Source: CAD feature listing. Evaluate the final solid. Frame: model axes, mm. Face numbers are marked on the shaded views. A direction names the side the tool comes from. Round coordinates to 2 decimals unless told otherwise and drop trailing zeros. Order: outer loops, then holes, each group sorted by start corner. A loop starts at its lowest first (then second) coordinate and runs counter-clockwise, first axis right, second up. Notation, with made-up numbers: M -39,70 L 17,70 A16 cw 17,79 Z; hole C 14,51 d6. An arc over 180 degrees is marked long. Use CSV: the item, a comma, the result in double quotes. Start each with the question number.
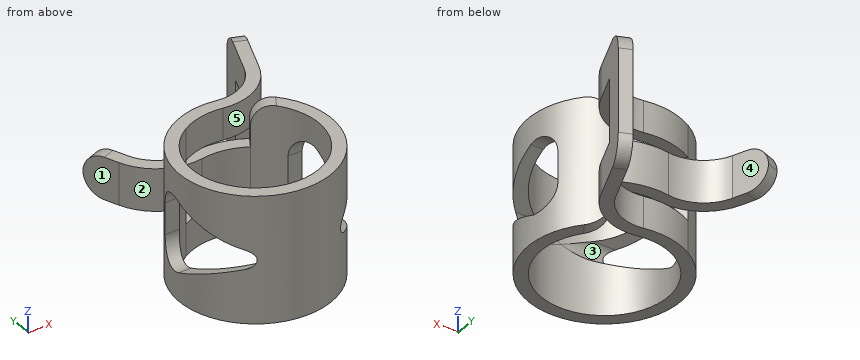
```python
from build123d import *

# Parameters (mm, degrees)
CYLINDER_SKETCH_R               = 3.6
CYLINDER_SKETCH_R_2             = 3
CYLINDER_EXTRUDE_DEPTH          = 3
CUT_SIDE_SLOTS_DEPTH            = 12.7
CUT_SLOT_IN_TOP_DEPTH           = 8.868926397
FEMALE_BASE_SKETCH_W            = 1.5
FEMALE_BASE_SKETCH_H            = 0.6
FEMALE_BASE_ANGLE               = 40.5
FEMALE_TRANSITION_SKETCH_W      = 1.5
FEMALE_TRANSITION_SKETCH_H      = 0.6
FEMALE_TRANSITION_REVOLVE_ANGLE = 78
FEMALE_LEVER_SKETCH_W           = 0.6
FEMALE_LEVER_SKETCH_H           = 1.5
FEMALE_LEVER_EXTRUDE_DEPTH      = 1.5
FEMALE_TOP_SKETCH_W             = 0.6
FEMALE_TOP_SKETCH_H             = 6
FEMALE_TOP_EXTRUDE_DEPTH        = 1.5
MALE_BASE_SKETCH_W              = 2
MALE_BASE_SKETCH_H              = 0.6
MALE_BASE_ANGLE                 = 40.5
MALE_TRANSITION_SKETCH_W        = 2
MALE_TRANSITION_SKETCH_H        = 0.6
MALE_TRANSITION_REVOLVE_ANGLE   = 78
MALE_LEVER_SKETCH_W             = 0.6
MALE_LEVER_SKETCH_H             = 2
MALE_LEVER_EXTRUDE_DEPTH        = 1.714285714
FILLETS_R                       = 1.016


with BuildPart() as part:
    # Cylinder Sketch → Cylinder Extrude (new, symmetric)
    with BuildSketch(Plane.XY):
        Circle(CYLINDER_SKETCH_R)
        Circle(CYLINDER_SKETCH_R_2, mode=Mode.SUBTRACT)
    extrude(amount=CYLINDER_EXTRUDE_DEPTH, both=True)

    # Side Slot Sketch → Cut Side Slots (cut, symmetric)
    with BuildSketch(Plane(origin=(0, 0, 0), x_dir=(0, 0, -1), z_dir=(1, 0, 0))):
        with BuildLine():
            Line((-0.75, 1.5), (0.75, 1.5))
            ThreePointArc((0.75, 1.5), (1.585525874, 1.049451102), (1.668161225, 0.103793027))
            Line((1.668161225, 0.103793027), (0.459080612, -2.698103486))
            ThreePointArc((0.459080612, -2.698103486), (0, -3), (-0.459080612, -2.698103486))
            Line((-0.459080612, -2.698103486), (-1.668161225, 0.103793027))
            ThreePointArc((-1.668161225, 0.103793027), (-1.585525874, 1.049451102), (-0.75, 1.5))
        make_face()
    extrude(amount=CUT_SIDE_SLOTS_DEPTH, both=True, mode=Mode.SUBTRACT)

    # Top Slot Sketch → Cut Slot in Top (cut, through all)
    with BuildSketch(Plane.XY.offset(3)):
        Polygon((-2.163098228, 3.6), (0, 0), (2.163098228, 3.6), align=None)
    extrude(amount=-CUT_SLOT_IN_TOP_DEPTH, mode=Mode.SUBTRACT)

    # Female Base Sketch → Female Base (revolve)
    with BuildSketch(Plane(origin=(0, 0, 0), x_dir=(0, 0, -1), z_dir=(0.8571673007021136, 0.515038074910052, 0))):
        with Locations((-2.25, 3.3)):
            Rectangle(FEMALE_BASE_SKETCH_W, FEMALE_BASE_SKETCH_H)
        with Locations((2.25, 3.3)):
            Rectangle(FEMALE_BASE_SKETCH_W, FEMALE_BASE_SKETCH_H)
    revolve(axis=Axis((0, 0, 0), (0, 0, -1)), revolution_arc=FEMALE_BASE_ANGLE)

    # Female Transition Sketch → Female Transition Revolve (revolve)
    with BuildSketch(Plane(origin=(0, 0, 0), x_dir=(0, 0, -1), z_dir=(0.9862856015372308, -0.16504760586068196, 0))):
        with Locations((2.25, 3.3)):
            Rectangle(FEMALE_TRANSITION_SKETCH_W, FEMALE_TRANSITION_SKETCH_H)
        with Locations((-2.25, 3.3)):
            Rectangle(FEMALE_TRANSITION_SKETCH_W, FEMALE_TRANSITION_SKETCH_H)
    revolve(axis=Axis((0.924266593, 5.523199369, 1.5), (0, 0, 1)), revolution_arc=FEMALE_TRANSITION_REVOLVE_ANGLE)

    # Female Lever Sketch → Female Lever Extrude (add)
    with BuildSketch(Plane(origin=(2.007556855, 5.096479986, 0), x_dir=(0.9304175679820241, -0.3665012267242986, 0), z_dir=(0.3665012267242986, 0.9304175679820241, 0))):
        with Locations((1.135694531, 2.25)):
            Rectangle(FEMALE_LEVER_SKETCH_W, FEMALE_LEVER_SKETCH_H)
        with Locations((1.135694531, -2.25)):
            Rectangle(FEMALE_LEVER_SKETCH_W, FEMALE_LEVER_SKETCH_H)
    extrude(amount=FEMALE_LEVER_EXTRUDE_DEPTH)

    # Female Top Sketch → Female Top Extrude (add)
    with BuildSketch(Plane(origin=(2.557308695, 6.492106338, 0), x_dir=(0.930417567982024, -0.3665012267242986, 0), z_dir=(0.3665012267242986, 0.9304175679820241, 0))):
        with Locations((1.135694531, 0)):
            Rectangle(FEMALE_TOP_SKETCH_W, FEMALE_TOP_SKETCH_H)
    extrude(amount=FEMALE_TOP_EXTRUDE_DEPTH)

    # Male Base Sketch → Male Base (revolve)
    with BuildSketch(Plane(origin=(0, 0, 0), x_dir=(0, 0, 1), z_dir=(-0.8571673007021136, 0.515038074910052, 0))):
        with Locations((0, 3.3)):
            Rectangle(MALE_BASE_SKETCH_W, MALE_BASE_SKETCH_H)
    revolve(axis=Axis((0, 0, 0), (0, 0, 1)), revolution_arc=MALE_BASE_ANGLE)

    # Male Transition Sketch → Male Transition Revolve (revolve)
    with BuildSketch(Plane(origin=(0, 0, 0), x_dir=(0, 0, 1), z_dir=(-0.9862856015372308, -0.16504760586068182, 0))):
        with Locations((0, 3.3)):
            Rectangle(MALE_TRANSITION_SKETCH_W, MALE_TRANSITION_SKETCH_H)
    revolve(axis=Axis((-0.924266593, 5.523199369, -1), (0, 0, -1)), revolution_arc=MALE_TRANSITION_REVOLVE_ANGLE)

    # Male Lever Sketch → Male Lever Extrude (add)
    with BuildSketch(Plane(origin=(-2.007556855, 5.096479986, 0), x_dir=(0.9304175679820241, 0.3665012267242986, 0), z_dir=(-0.3665012267242986, 0.9304175679820241, 0))):
        with Locations((-1.135694531, 0)):
            Rectangle(MALE_LEVER_SKETCH_W, MALE_LEVER_SKETCH_H)
    extrude(amount=MALE_LEVER_EXTRUDE_DEPTH)

    # Fillets
    # the kernel refuses this fillet: 1.016 mm, written as the material it takes off along each edge
    with BuildSketch(Plane(origin=(0.236917514, 0.394296958, -3), x_dir=(0.8571673007021136, -0.5150380749100519, 0), z_dir=(0.515038074910052, 0.8571673007021137, 0))) as fillets_piece_1_section:
        with BuildLine():
            CenterArc((FILLETS_R, -FILLETS_R), FILLETS_R, 90, 90)
            Line((0, -FILLETS_R), (0, 0))
            Line((0, 0), (FILLETS_R, 0))
        make_face()
    fillets_piece_1 = extrude(amount=5.68, mode=Mode.PRIVATE)
    fillets_piece_1 = fillets_piece_1 & Plane(origin=(0, 0, -2.773460416), x_dir=(1, 0, 0), z_dir=(0, 0, 1)) * Cylinder(3.6, 16, mode=Mode.PRIVATE)
    add(fillets_piece_1, mode=Mode.SUBTRACT)
    with BuildSketch(Plane(origin=(0.236917514, 0.394296958, 3), x_dir=(0, 0, -1), z_dir=(0.515038074910052, 0.8571673007021137, 0))) as fillets_piece_2_section:
        with BuildLine():
            CenterArc((FILLETS_R, -FILLETS_R), FILLETS_R, 90, 90)
            Line((0, -FILLETS_R), (0, 0))
            Line((0, 0), (FILLETS_R, 0))
        make_face()
    fillets_piece_2 = extrude(amount=5.68, mode=Mode.PRIVATE)
    fillets_piece_2 = fillets_piece_2 & Plane(origin=(0, 0, 2.773461153), x_dir=(1, 0, 0), z_dir=(0, 0, 1)) * Cylinder(3.6, 16, mode=Mode.PRIVATE)
    add(fillets_piece_2, mode=Mode.SUBTRACT)
    with BuildSketch(Plane(origin=(-6.334900709, 5.234384608, 1), x_dir=(0.3665012267242986, -0.930417567982024, 0), z_dir=(0.9304175679820241, 0.3665012267242986, 0)), Plane(origin=(-1.050128923, 7.316111576, -1), x_dir=(0.3665012267242985, -0.930417567982024, 0), z_dir=(-0.9304175679820241, -0.3665012267242986, 0))) as fillets_piece_3:
        with BuildLine():
            CenterArc((FILLETS_R, FILLETS_R), FILLETS_R, 180, 90)
            Line((0, FILLETS_R), (0, 0))
            Line((0, 0), (FILLETS_R, 0))
        make_face()
    extrude(amount=5.68, mode=Mode.SUBTRACT)
    with BuildSketch(Plane(origin=(1.521344786, 8.512362735, -3), x_dir=(-0.3665012267242986, -0.930417567982024, 0), z_dir=(0.9304175679820241, -0.3665012267242986, 0)), Plane(origin=(6.806116572, 6.430635767, 3), x_dir=(-0.3665012267242985, -0.930417567982024, 0), z_dir=(-0.9304175679820241, 0.3665012267242986, 0))) as fillets_piece_4:
        with BuildLine():
            CenterArc((FILLETS_R, -FILLETS_R), FILLETS_R, 90, 90)
            Line((0, -FILLETS_R), (0, 0))
            Line((0, 0), (FILLETS_R, 0))
        make_face()
    extrude(amount=5.68, mode=Mode.SUBTRACT)


solid = part.part
```
(1) Reachability of the marked faces 3, 4 and 5 from +Z, -Z, +X, -X, +Y, -Y: full face, straight path, thin tool, end or side. Return the list, or none.
(2) Line query: line 1 along Y through (x, z) = (2, -2.25); line 2 along Y through (x, z) = (0, -0.25); line 3 along Y through (x, z) = (0, 1.25). Output: solid intervals per line, ascending.
(3) Section B-B on z = -1.25. Return loops of the section in (x, y).
(4) Section A-A on x = -0.25. Return loops of the section in (y, z).
(5) Section C-C on x = -2. Return loops of the section in (y, z).
(6) Draft query along Z for the marked faces 1 and 2. Return one class per face: pulls with the +Z half, pulls with the -Z half, needs draft (parallel to the pull), parting line crosses it, or undercut.
(7) Contact query for flat-ended pins moving along their axis: P1, Ø3.5, axis at x = 0, y = 0, coming from the +Z side; P2, Ø2, axis at y = -1, z = -2, coming from the -X side; P3, Ø2, axis at x = 3, z = 0.5, coming from the -Y side. Output: stop coordinate, or through.
Results below:
1,face 3,"+X, -X"
1,face 4,"+Z, -Z, +Y"
1,face 5,"+Z"
2,line 1,"y = -2.99 to -2.24, 2.24 to 2.99, 3.16 to 3.84"
2,line 2,"y = -3.6 to -3, 3 to 3.6"
2,line 3,"y = -3.6 to -3"
3,outline,"M -3.49,-0.87 A3.6 ccw 3.49,-0.87 L 2.87,-0.87 A3 cw -2.87,-0.87 Z; M -3.33,1.37 L -2.67,1.37 A3 cw -1.55,2.57 L -1.85,3.09 A3.6 ccw Z; M 1.55,2.57 A3 cw 2.67,1.37 L 3.33,1.37 A3.6 ccw 1.85,3.09 Z; M 3.33,6.19 L 3.89,5.97 L 4.44,7.36 L 3.88,7.58 Z"
4,outline,"M -3.59,-3 L -2.99,-3 L -2.99,-0.1 A0.5 cw -2.99,0.1 L -2.99,3 L -3.59,3 Z; M 2.99,-3 L 3.59,-3 L 3.59,-1.5 L 2.99,-1.5 Z; M 2.99,-1 L 3.59,-1 L 3.59,1 L 2.99,1 Z; M 2.99,1.5 L 3.59,1.5 L 3.59,3 L 2.99,3 Z"
5,outline,"M -2.99,-3 L -2.24,-3 L -2.24,-0.66 L -2.7,-0.46 A0.5 cw -2.99,-0.08 Z; M -2.99,0.08 A0.5 cw -2.7,0.46 L -2.24,0.66 L -2.24,3 L -2.99,3 Z; M 2.24,-3 L 2.99,-3 L 2.99,3 L 2.24,3 Z; M 3.16,-1 L 3.84,-1 L 3.84,1 L 3.16,1 Z"
6,face 1,"needs draft"
6,face 2,"undercut"
7,P1,"passes through"
7,P2,"stops at x = -3.6"
7,P3,"stops at y = -2.99"
